from build123d import *

# Parameters (mm, degrees)
MAIN_EXTRUSION_DEPTH = 20
WHOLES_R             = 1.5
WHOLE_REMOVAL_DEPTH  = 9


with BuildPart() as part:
    # Main → Main Extrusion (new body)
    with BuildSketch(Plane.XY):
        Polygon((0, 17), (0, -17), (2, -17), (2, -7), (8, -7), (8, -2.5), (6, -2.5), (6, -5), (2, -5), (2, 5), (6, 5), (6, 2.5), (8, 2.5), (8, 7), (2, 7), (2, 17), align=None)
    extrude(amount=MAIN_EXTRUSION_DEPTH)

    # Wholes → Whole Removal (cut, through all)
    with BuildSketch(Plane.ZY):
        with Locations((5, 12.5)):
            Circle(WHOLES_R)
        with Locations((5, -12.5)):
            Circle(WHOLES_R)
        with Locations((15, -12.5)):
            Circle(WHOLES_R)
        with Locations((15, 12.5)):
            Circle(WHOLES_R)
    extrude(amount=-WHOLE_REMOVAL_DEPTH, mode=Mode.SUBTRACT)


solid = part.part
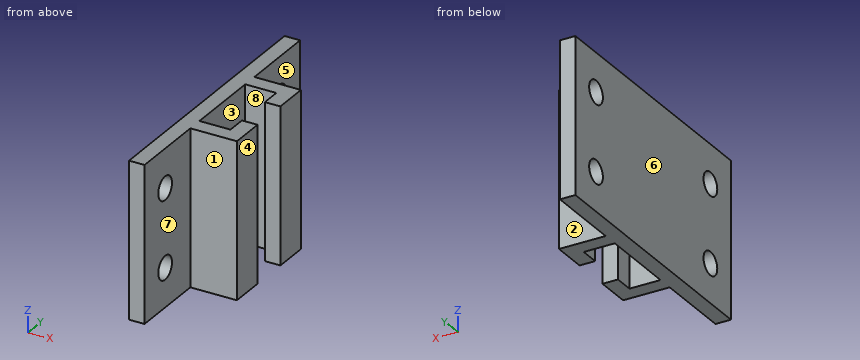
Source: CAD feature listing. Evaluate the final solid. Frame: model axes, mm. Face numbers are marked on the shaded views. A direction names the side the tool comes from. Coordinates: 2 decimals unless noted, no trailing zeros. Order: outer loops, then holes, each group sorted by start corner. A loop starts at its lowest first (then second) coordinate and runs counter-clockwise, first axis right, second up. Notation, with made-up numbers: M 10.5,36.25 L 14.5,36.25 A24 cw 14.5,75.25 Z; hole C 72,53 d2. An arc over 180 degrees is marked long. Write each question's results on one line, items separated by ' | '. Start each with the question number.
Item 1: Line query: probe 1 along Y at (x, z) = (0.55, 5); probe 2 along X at (y, z) = (3, 9); probe 3 along Y at (x, z) = (4.5, 18). Output: solid intervals per line, ascending.
Item 2: Set-up query: the marked faces 5, 6, 7 and 8. Return all of +Z, -Z, +X, -X, +Y, -Y with unobstructed straight access to the full face (end or side cutting, diameter ignored); none if empty.
Item 3: First-contact query: pin 1 Ø1.8 at (y, z) = (-12.5, 15) entering from -X; pin 2 Ø3 at (y, z) = (-13.5, 9.5) entering from +X; pin 3 Ø1.8 at (x, z) = (4, 12.5) entering from +Y; pin 4 Ø2 at (x, z) = (4.5, 9) entering from -Y. Flat tips, straight axial feed; report the tip coordinate or a pass-through.
Item 4: Cut plane C-C (z = 5). Return loops of the section in (x, y), and give its area (3 significant figures).
Item 5: Cut plane B-B (x = 5.25). Return loops of the section in (y, z), and give its area (3 significant figures).
Item 6: Draft query along Y for the marked faces 1, 2, 3 and 4. Return one class per face: pulls with the +Y half, pulls with the -Y half, needs draft (parallel to the pull), parting line crosses it, or undercut.
Item 7: Cut plane A-A (y = -12.5). Return loops of the section in (x, z).
Item 8: Cut plane D-D (z = 13). Return loops of the section in (x, y).
Checked values:
1) probe 1: y = -17 to -14, -11 to 11, 14 to 17 | probe 2: x = 0 to 2, 6 to 8 | probe 3: y = -7 to -5, 5 to 7
2) face 5: +Z, -Z, +X, +Y | face 6: +Z, -Z, -X, +Y, -Y | face 7: +Z, -Z, +X, -Y | face 8: +Z, -Z
3) pin 1: passes through | pin 2: stops at x = 2 | pin 3: stops at y = 7 | pin 4: stops at y = -7
4) outline: M 0,-17 L 2,-17 L 2,-14 L 0,-14 Z; M 0,-11 L 2,-11 L 2,-7 L 8,-7 L 8,-2.5 L 6,-2.5 L 6,-5 L 2,-5 L 2,5 L 6,5 L 6,2.5 L 8,2.5 L 8,7 L 2,7 L 2,11 L 0,11 Z; M 0,14 L 2,14 L 2,17 L 0,17 Z | area: 90.0 mm2
5) outline: M -7,0 L -5,0 L -5,20 L -7,20 Z; M 5,0 L 7,0 L 7,20 L 5,20 Z | area: 80.0 mm2
6) face 1: pulls with the -Y half | face 2: pulls with the +Y half | face 3: undercut | face 4: needs draft
7) outline: M 0,0 L 2,0 L 2,3.5 L 0,3.5 Z; M 0,6.5 L 2,6.5 L 2,13.5 L 0,13.5 Z; M 0,16.5 L 2,16.5 L 2,20 L 0,20 Z
8) outline: M 0,-17 L 2,-17 L 2,-7 L 8,-7 L 8,-2.5 L 6,-2.5 L 6,-5 L 2,-5 L 2,5 L 6,5 L 6,2.5 L 8,2.5 L 8,7 L 2,7 L 2,17 L 0,17 Z
